Read the model definition and answer for the solid it produces. Units are mm, in the model's axes. Face numbers are marked on the shaded views. A direction names the side the tool comes from. Give positions to 0.01 mm unless a question says otherwise; leave off trailing zeros. Order: outer loops, then holes, each group sorted by start corner. A loop starts at its lowest first (then second) coordinate and runs counter-clockwise, first axis right, second up.
Item 1: Find the intervals of material crossed by line 1 along X through (y, z) = (9, 2.25); line 2 along X through (y, z) = (19, 3); line 3 along X through (y, z) = (3.5, 3.75), in increasing order.
Item 2: Given pin 1 Ø3 at (x, y) = (21.24, 3.36) entering from -Z; pin 2 Ø5 at (x, y) = (-4.5, 26) entering from -Z; pin 3 Ø2 at (y, z) = (-23, 4) entering from +X; pin 4 Ø8 at (x, y) = (17.68, 17.68) entering from -Z, each flat-ended and moving along its own axis, determine where each tip first touches the part or whether it passes through.
Item 3: A cutting plane is placed at A-A (x = 0). Write down the section's boundary in (y, z).
Item 4: A cutting plane is placed at C-C (z = 1.25). State how many separate pieces and enclosed holes the cut face has, plus the area to 3 significant figures.
Item 5: The mould has two halves that part along X. Classify the marked faces 1, 2 and 3: +X half, -X half, draft (parallel to the pull), parting line (faces both ways), or undercut.
Item 6: A cutting plane is placed at D-D (y = 28). Write down the section's boundary in (x, z).
Item 7: Which of the six approach directions +Z, -Z, +X, -X, +Y, -Y give full straight-line access (tool end or side, diameter ignored) to the marked faces 4 and 5?
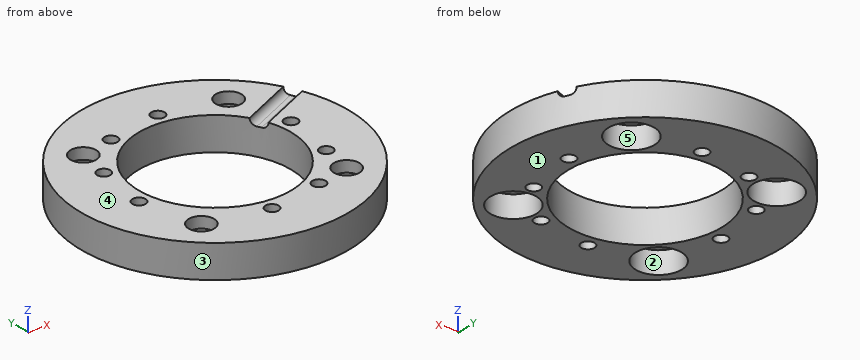
from build123d import *

# Parameters (mm, degrees)
SKETCH1_R           = 32.5
SKETCH1_R_2         = 3.1
SKETCH1_R_3         = 18.5
BOSS_EXTRUDE2_DEPTH = 8
SKETCH1_6_R         = 18.5
SKETCH1_6_R_2       = 5.55
SKETCH1_6_R_3       = 3.1
CUT_EXTRUDE2_DEPTH  = 5.3
SKETCH2_R           = 1.6
CUT_EXTRUDE3_DEPTH  = 10
CUT_EXTRUDE4_DEPTH  = 1.5
FILLET1_R           = 1.5


with BuildPart() as part:
    # Sketch1 → Boss-Extrude2 (new body)
    with BuildSketch(Plane.XY):
        Circle(SKETCH1_R)
        with Locations((17.67766953, 17.67766953)):
            Circle(SKETCH1_R_2, mode=Mode.SUBTRACT)
        with Locations((17.67766953, -17.67766953)):
            Circle(SKETCH1_R_2, mode=Mode.SUBTRACT)
        with Locations((-17.67766953, -17.67766953)):
            Circle(SKETCH1_R_2, mode=Mode.SUBTRACT)
        with Locations((-17.67766953, 17.67766953)):
            Circle(SKETCH1_R_2, mode=Mode.SUBTRACT)
        Circle(SKETCH1_R_3, mode=Mode.SUBTRACT)
    extrude(amount=BOSS_EXTRUDE2_DEPTH)

    # Sketch1<6> → Cut-Extrude2 (cut)
    # profile 1 of 8: a face of its own
    with BuildSketch(Plane.XY):
        Circle(SKETCH1_6_R)
    # profile 2 of 8: a face of its own
    with BuildSketch(Plane.XY):
        with Locations((17.67766953, 17.67766953)):
            Circle(SKETCH1_6_R_2)
        with Locations((17.67766953, 17.67766953)):
            Circle(SKETCH1_6_R_3, mode=Mode.SUBTRACT)
    # profile 3 of 8: a face of its own
    with BuildSketch(Plane.XY):
        Circle(SKETCH1_6_R)
    # profile 4 of 8: a face of its own
    with BuildSketch(Plane.XY):
        with Locations((17.67766953, -17.67766953)):
            Circle(SKETCH1_6_R_2)
        with Locations((17.67766953, -17.67766953)):
            Circle(SKETCH1_6_R_3, mode=Mode.SUBTRACT)
    # profile 5 of 8: a face of its own
    with BuildSketch(Plane.XY):
        Circle(SKETCH1_6_R)
    # profile 6 of 8: a face of its own
    with BuildSketch(Plane.XY):
        with Locations((-17.67766953, -17.67766953)):
            Circle(SKETCH1_6_R_2)
        with Locations((-17.67766953, -17.67766953)):
            Circle(SKETCH1_6_R_3, mode=Mode.SUBTRACT)
    # profile 7 of 8: a face of its own
    with BuildSketch(Plane.XY):
        Circle(SKETCH1_6_R)
    # profile 8 of 8: a face of its own
    with BuildSketch(Plane.XY):
        with Locations((-17.67766953, 17.67766953)):
            Circle(SKETCH1_6_R_2)
        with Locations((-17.67766953, 17.67766953)):
            Circle(SKETCH1_6_R_3, mode=Mode.SUBTRACT)
    extrude(amount=CUT_EXTRUDE2_DEPTH, mode=Mode.SUBTRACT)

    # Sketch2 → Cut-Extrude3 (cut)
    with BuildSketch(Plane(origin=(0, 0, 0), x_dir=(-1, 0, 0), z_dir=(0, 0, -1))):
        with Locations((9.760795744, 19.15664027)):
            Circle(SKETCH2_R)
        with Locations((19.15664027, 9.760795744)):
            Circle(SKETCH2_R)
        with Locations((21.235299323, -3.363340998)):
            Circle(SKETCH2_R)
        with Locations((3.363340998, -21.235299323)):
            Circle(SKETCH2_R)
        with Locations((-9.760795744, -19.15664027)):
            Circle(SKETCH2_R)
        with Locations((-19.15664027, -9.760795744)):
            Circle(SKETCH2_R)
        with Locations((-21.235299323, 3.363340998)):
            Circle(SKETCH2_R)
        with Locations((-3.363340998, 21.235299323)):
            Circle(SKETCH2_R)
    extrude(amount=-CUT_EXTRUDE3_DEPTH, mode=Mode.SUBTRACT)

    # Sketch4 → Cut-Extrude4 (cut)
    with BuildSketch(Plane.XY.offset(8)):
        Polygon((14.516655151, 4.273958731), (32.787564304, 12.408691592), (31.160617731, 16.062873423), (12.889708578, 7.928140561), align=None)
    extrude(amount=-CUT_EXTRUDE4_DEPTH, mode=Mode.SUBTRACT)

    # Fillet1
    fillet1_edges = [part.edges().sort_by_distance(p)[0] for p in [
        (22.404274162, 12.164298088, 6.5),
        (24.031220735, 8.510116257, 6.5),
    ]]
    fillet(fillet1_edges, radius=FILLET1_R - 0.0001)  # a hair under: the kernel refuses the full size


solid = part.part
Response values:
1. line 1: x = -31.23 to -20.56, -17.75 to -16.16, 16.16 to 31.23
1. line 2: x = -26.37 to -23.07, -12.29 to -11.35, -8.17 to 12.29, 23.07 to 26.37
1. line 3: x = -32.31 to -18.17, 18.17 to 19.64, 22.83 to 32.31
2. pin 1: passes through
2. pin 2: stops at z = 0
2. pin 3: stops at x = 23.92
2. pin 4: stops at z = 5.3
3. outline: (-32.5, 0) - (-18.5, 0) - (-18.5, 8) - (-32.5, 8) - close; (18.5, 0) - (32.5, 0) - (32.5, 8) - (18.5, 8) - close
4. separate pieces: 1
4. enclosed holes: 13
4. area: 1,790 mm2
5. face 1: draft
5. face 2: undercut
5. face 3: parting line
6. outline: (-16.5, 0) - (16.5, 0) - (16.5, 8) - (-16.5, 8) - close
7. face 4: +Z, +X, -X, +Y, -Y
7. face 5: -Z
